Work out the finished part from the listing and answer in its coordinate system (mm). Give positions to 0.01 mm unless a question says otherwise; leave off trailing zeros. Write each loop counter-clockwise with the first axis right and the second up, starting at its lowest first coordinate (ties: lowest second). Pieces come first, ordered by that corner, then holes.
1) Find section B-B (x = -1.5). Determine the outline of the cut face in (y, z).
2) Find section C-C (z = 5.5). Determine the outline of the cut face in (x, y).
3) Find section A-A (y = 0). Determine the outline of the cut face in (x, z).
4) Given pin 1 Ø4 at (x, z) = (2.5, 1) entering from -Y; pin 2 Ø4 at (x, z) = (0, 2) entering from -Y, each flat-ended and moving along its own axis, determine where each tip first touches the part or whether it passes through.
5) Straight lines are drawn through the part: probe 1 along Y at (x, z) = (0, 7); probe 2 along Y at (x, z) = (-1.75, 8); probe 3 along Z at (x, y) = (-6, 2). For each, find the intervals that lie inside material, in ascending order.
6) Find section D-D (y = 4.75). Determine the outline of the cut face in (x, z).
7) Determine the mould class of faces 1 (the face through (5.96, 1.88, 6.46)), 2 (the face through (-4, -5, 4)), 3 (the face through (0.54, -2.44, 4.44)), 4 (the face through (7.794, 0, 2)) for opening direction X: pulls with the +X half, pulls with the -X half, needs draft (parallel to the pull), parting line crosses it, or undercut.
```python
from build123d import *

# Parameters (mm, degrees)
F2_DEPTH = 4
F1_R     = 6.25
F3_DEPTH = 9
F5_D     = 5


with BuildPart() as f2:
    # F0 (on Top) → F2 (new body)
    with BuildSketch(Plane.XY):
        Polygon((-7.794229, 4.5), (-7.794229, -4.5), (0, -9), (7.794229, -4.5), (7.794229, 4.5), (0, 9), align=None)
    extrude(amount=F2_DEPTH)

    # F1 (on Top) → F3 (join)
    with BuildSketch(Plane.XY):
        Circle(F1_R)
    extrude(amount=F3_DEPTH)

    # F5 (through all)
    with Locations(Plane.XY.offset(9)):
        with Locations((0, 0)):
            Hole(F5_D / 2)


solid = f2.part
```
Results:
1. outline: (-8.13, 0) - (-2, 0) - (-2, 9) - (-6.07, 9) - (-6.07, 4) - (-8.13, 4) - close; (2, 0) - (8.13, 0) - (8.13, 4) - (6.07, 4) - (6.07, 9) - (2, 9) - close
2. outline: circle Ø12.5 at (0, 0); hole circle Ø5 at (0, 0)
3. outline: (-7.79, 0) - (-2.5, 0) - (-2.5, 9) - (-6.25, 9) - (-6.25, 4) - (-7.79, 4) - close; (2.5, 0) - (7.79, 0) - (7.79, 4) - (6.25, 4) - (6.25, 9) - (2.5, 9) - close
4. pin 1: stops at y = -8.71
4. pin 2: stops at y = -9
5. probe 1: y = -6.25 to -2.5, 2.5 to 6.25
5. probe 2: y = -6 to -1.79, 1.79 to 6
5. probe 3: z = 0 to 4
6. outline: (-7.36, 0) - (7.36, 0) - (7.36, 4) - (4.06, 4) - (4.06, 9) - (-4.06, 9) - (-4.06, 4) - (-7.36, 4) - close
7. face 1: parting line crosses it
7. face 2: needs draft
7. face 3: undercut
7. face 4: pulls with the +X half
